from build123d import *

# Parameters (mm, degrees)
SKETCH1_W             = 63.5
SKETCH1_H             = 6.35
BOSS_EXTRUDE1_DEPTH   = 3.175
F_6_CLEARANCE_HOLE1_D = 3.7973
SKETCH7_W             = 17.4625
SKETCH7_H             = 27.78125
BOSS_EXTRUDE2_DEPTH   = 3.175
SKETCH9_W             = 3.175
SKETCH9_H             = 20.6375
BOSS_EXTRUDE3_DEPTH   = 44.45
M3_CLEARANCE_HOLE1_D  = 3.4
SKETCH14_W            = 20.6375
SKETCH14_H            = 6.35
BOSS_EXTRUDE4_DEPTH   = 3.175
FILLET3_R             = 2.38125
M3_CLEARANCE_HOLE2_D  = 3.4
MIRROR1_START         = -8.73125
MIRROR1_OUTLINE_R     = 1.7
MIRROR1_DEPTH         = 3.175


# Read off the part's stored shape, not the designer's step: Mirror1
with BuildPart() as part:
    # Sketch1 → Boss-Extrude1 (new body)
    with BuildSketch(Plane(origin=(0, 0, 0), x_dir=(1, 0, 0), z_dir=(0, 1, 0))):
        with Locations((0, -3.175)):
            Rectangle(SKETCH1_W, SKETCH1_H)
        with Locations((0, 3.175)):
            Rectangle(SKETCH1_W, SKETCH1_H)
    extrude(amount=BOSS_EXTRUDE1_DEPTH)

    # #6 Clearance Hole1 (through all)
    with Locations(Plane(origin=(0, 0, 0), x_dir=(-1, 0, 0), z_dir=(0, -1, 0))):
        with Locations((25.4, 0), (-25.4, 0)):
            Hole(F_6_CLEARANCE_HOLE1_D / 2)

    # Sketch7 → Boss-Extrude2 (add)
    with BuildSketch(Plane.XZ):
        with Locations((0, -7.540625)):
            Rectangle(SKETCH7_W, SKETCH7_H)
    extrude(amount=-BOSS_EXTRUDE2_DEPTH)

    # Sketch9 → Boss-Extrude3 (add)
    with BuildSketch(Plane.XZ):
        with Locations((7.14375, -3.96875)):
            Rectangle(SKETCH9_W, SKETCH9_H)
        with Locations((-7.14375, -3.96875)):
            Rectangle(SKETCH9_W, SKETCH9_H)
    extrude(amount=-BOSS_EXTRUDE3_DEPTH)

    # M3 Clearance Hole1 (through all)
    with Locations(Plane(origin=(8.73125, 0, 0), x_dir=(0, 0, -1), z_dir=(1, 0, 0))):
        with Locations((0.79375, 19.84375), (11.90625, 42.06875)):
            Hole(M3_CLEARANCE_HOLE1_D / 2)

    # Sketch14 → Boss-Extrude4 (add)
    with BuildSketch(Plane(origin=(8.73125, 0, 0), x_dir=(0, 0, -1), z_dir=(1, 0, 0))):
        with Locations((3.96875, 47.625)):
            Rectangle(SKETCH14_W, SKETCH14_H)
        Polygon((14.2875, 50.8), (14.2875, 44.45), (14.2875, 38.89375), (20.6375, 38.89375), (20.6375, 50.8), align=None)
    extrude(amount=-BOSS_EXTRUDE4_DEPTH)

    # Fillet3
    fillet3_edges = [part.edges().sort_by_distance(p)[0] for p in [
        (7.14375, 50.8, -20.6375),
        (7.14375, 38.89375, -20.6375),
        (7.14375, 38.89375, -14.2875),
    ]]
    fillet(fillet3_edges, radius=FILLET3_R)

    # M3 Clearance Hole2 (through all)
    with Locations(Plane(origin=(8.73125, 0, 0), x_dir=(0, 0, -1), z_dir=(1, 0, 0))):
        with Locations((17.4625, 47.625)):
            Hole(M3_CLEARANCE_HOLE2_D / 2)

    # Mirror1 outline → Mirror1 (add)
    with BuildSketch(Plane.YZ.offset(MIRROR1_START)):
        with BuildLine():
            ThreePointArc((48.41875, -20.6375), (50.102548023, -19.940048023), (50.8, -18.25625))
            Line((50.8, -18.25625), (50.8, 6.35))
            Line((50.8, 6.35), (44.45, 6.35))
            Line((44.45, 6.35), (44.45, -14.2875))
            Line((44.45, -14.2875), (38.89375, -14.2875))
            Line((38.89375, -14.2875), (38.89375, -18.25625))
            ThreePointArc((38.89375, -18.25625), (39.591201977, -19.940048023), (41.275, -20.6375))
            Line((41.275, -20.6375), (48.41875, -20.6375))
        make_face()
        with Locations((47.625, -17.4625)):
            Circle(MIRROR1_OUTLINE_R, mode=Mode.SUBTRACT)
    extrude(amount=MIRROR1_DEPTH)


solid = part.part
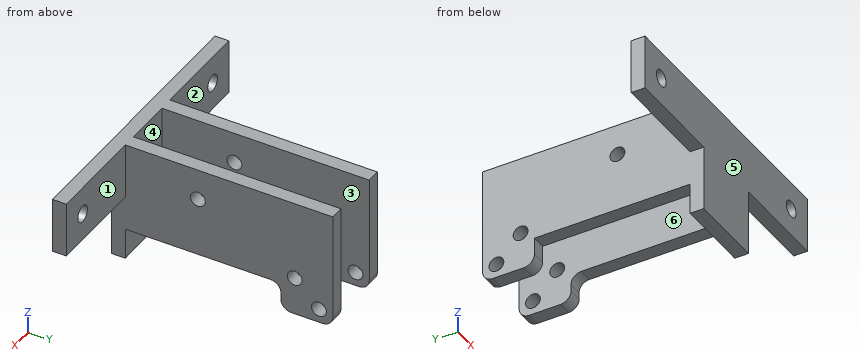
Source: CAD feature listing. Evaluate the final solid. Frame: model axes, mm. Face numbers are marked on the shaded views. A direction names the side the tool comes from. Give positions to 0.01 mm unless a question says otherwise; leave off trailing zeros. Write each loop counter-clockwise with the first axis right and the second up, starting at its lowest first coordinate (ties: lowest second). Pieces come first, ordered by that corner, then holes. Notation, with made-up numbers: M 4,-12 L 30,-12 A24 cw 30,4 Z; hole C 87.5,32 d6. An arc over 180 degrees is marked long. Return JSON: item names as keys, results as strings. Group by question number.
1) Ray query, L1, parallel to X at y = 35, z = -2.5; L2, parallel to Y at x = -0.5, z = 0.5 (3 decimals); L3, parallel to Z at x = 25, y = 2. Return the intervals inside material, ascending.
2) Cut plane D-D, the plane x = 7.5. Give the number of separate pieces and of enclosed holes in the cut face, then the cut area to 3 significant figures.
3) Draft query along X for the marked faces 5 and 6. Return one class per face: released by +X, released by -X, zero draft, split by the parting line, or undercut.
4) Cut plane B-B, the plane y = 5.5. Output: boundary loops of the cut face in (x, z).
5) Cut plane A-A, the plane x = 25.4. Output: boundary loops of the cut face in (y, z) (3 decimals), then the cut area to 3 significant figures.
6) First-contact query: pin 1 Ø1 at (x, z) = (-0.5, -9.5) entering from +Y (3 decimals); pin 2 Ø4 at (y, z) = (15.5, 2) entering from -X; pin 3 Ø4 at (y, z) = (47.62, -17.46) entering from +X; pin 4 Ø2.5 at (x, z) = (-25.4, 0) entering from -Y. Flat tips, straight axial feed; report the tip coordinate or a pass-through.
7) Set-up query: the marked faces 1, 2, 3 and 4. Return all of +Z, -Z, +X, -X, +Y, -Y with unobstructed straight access to the full face (end or side cutting, diameter ignored); none if empty.
8) Cut plane C-C, the plane z = -8.25. Output: boundary loops of the cut face in (x, y) (3 decimals).
Data:
{
 "1": {"L1": "x = -8.73 to -5.56, 5.56 to 8.73", "L2": "y = 0 to 3.175", "L3": "z = -6.35 to -1.86, 1.86 to 6.35"},
 "2": {"separate pieces": "1", "enclosed holes": "3", "area": "1,120 mm²"},
 "3": {"face 5": "zero draft", "face 6": "undercut"},
 "4": {"outline": "M -8.73,-14.29 L -5.56,-14.29 L -5.56,6.35 L -8.73,6.35 Z; M 5.56,-14.29 L 8.73,-14.29 L 8.73,6.35 L 5.56,6.35 Z"},
 "5": {"outline": "M 0,-6.35 L 3.175,-6.35 L 3.175,-1.899 L 0,-1.899 Z; M 0,1.899 L 3.175,1.899 L 3.175,6.35 L 0,6.35 Z", "area": "28.3 mm²"},
 "6": {"pin 1": "stops at y = 3.175", "pin 2": "stops at x = -8.73", "pin 3": "stops at x = 8.73", "pin 4": "passes through"},
 "7": {"face 1": "+Z, -Z, +X, +Y", "face 2": "+Z, -Z, -X, +Y", "face 3": "+Z, -Z, +Y", "face 4": "-Z"},
 "8": {"outline": "M -8.731,0 L 8.731,0 L 8.731,50.8 L 5.556,50.8 L 5.556,3.175 L -5.556,3.175 L -5.556,50.8 L -8.731,50.8 Z"}
}
